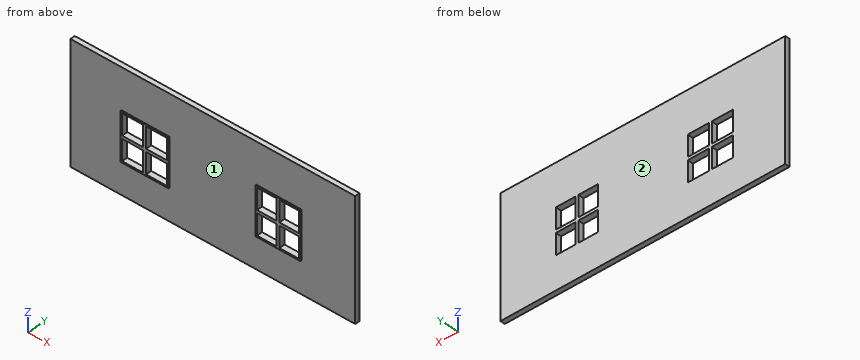
```python
from build123d import *

# Parameters (mm, degrees)
F0_W      = 95
F0_H      = 1.6
F1_DEPTH  = 40
F2_W      = 15
F2_H      = 15
F2_W_2    = 14
F3_DEPTH  = 25
F4_W      = 16
F4_H      = 16
F4_W_2    = 15
F4_H_2    = 15
F4_W_3    = 14
F5_DEPTH  = 0.3
F6_W      = 1
F6_H      = 1.9
F7_DEPTH  = 15
F11_DEPTH = 15
F10_W     = 1.9
F10_H     = 1
F12_DEPTH = 14


with BuildPart() as f1:
    # F0 (on Top) → F1 (new body)
    with BuildSketch(Plane.XY):
        Rectangle(F0_W, F0_H)
    extrude(amount=F1_DEPTH)

    # F2 (on face) → F3 (cut)
    with BuildSketch(Plane.XZ.offset(0.8)):
        with Locations((-22.5, 18.5)):
            Rectangle(F2_W, F2_H)
        with Locations((22, 18.5)):
            Rectangle(F2_W_2, F2_H)
    extrude(amount=-F3_DEPTH, mode=Mode.SUBTRACT)

    # F4 (on face) → F5 (join)
    with BuildSketch(Plane.XZ.offset(0.8)):
        with Locations((-22.5, 18.5)):
            Rectangle(F4_W, F4_H)
        with Locations((-22.5, 18.5)):
            Rectangle(F4_W_2, F4_H_2, mode=Mode.SUBTRACT)
        with Locations((22, 18.5)):
            Rectangle(F4_W_2, F4_H)
        with Locations((22, 18.5)):
            Rectangle(F4_W_3, F4_H_2, mode=Mode.SUBTRACT)
    extrude(amount=F5_DEPTH)

    # F6 (on face) → F7 (join, through all)
    with BuildSketch(Plane.XY.offset(11)):
        with Locations((22, -0.15)):
            Rectangle(F6_W, F6_H)
        with Locations((-22.5, -0.15)):
            Rectangle(F6_W, F6_H)
    extrude(amount=F7_DEPTH)

    # F9 (on face) → F11 (join, through all)
    with BuildSketch(Plane(origin=(-15, 0, 0), x_dir=(0, -1, 0), z_dir=(-1, 0, 0))):
        Polygon((-0.8, 18), (0.8, 18), (1.1, 18), (1.1, 19), (-0.8, 19), align=None)
    extrude(amount=F11_DEPTH)

    # F10 (on face) → F12 (join, through all)
    with BuildSketch(Plane(origin=(29, 0, 0), x_dir=(0, -1, 0), z_dir=(-1, 0, 0))):
        with Locations((0.15, 18.5)):
            Rectangle(F10_W, F10_H)
    extrude(amount=F12_DEPTH)


solid = f1.part
```
Read the model definition and answer for the solid it produces. Units are mm, in the model's axes. Face numbers are marked on the shaded views. Give positions to 0.01 mm unless a question says otherwise; leave off trailing zeros. Write each loop counter-clockwise with the first axis right and the second up, starting at its lowest first coordinate (ties: lowest second). Pieces come first, ordered by that corner, then holes. Notation, with made-up numbers: M 39,69 L 43,69 A22 ccw 43,93 Z; hole C -8.5,-6 d6. An arc over 180 degrees is marked long. Put each result on its own line as item: value. Start each with the question number.
1. The part is cut by section C-C, the plane y = 0.1. Give the number of separate pieces and of enclosed holes in the cut face, and give its area (3 significant figures).
2. Consider line 1 along Z through (x, y) = (19, 0.25); line 2 along X through (y, z) = (0.7, 22.5); line 3 along Y through (x, z) = (-41, 27). Determine where each line is inside the solid, lowest interval first.
3. For a pull along X with two mould halves and no side action, classify the marked faces 1 and 2 as released by +X, released by -X, zero draft, split by the parting line, or undercut.
4. The part is cut by section D-D, the plane x = 5.5. Give the vertices of the cut face in (y, z).
5. The part is cut by section B-B, the plane x = -18.5. Give the vertices of the cut face in (y, z), and give its area (3 significant figures).
6. The part is cut by section A-A, the plane z = 15.5. Give the vertices of the cut face in (x, y).
Final values:
1. separate pieces: 1
1. enclosed holes: 8
1. area: 3,420 mm²
2. line 1: z = 0 to 11, 18 to 19, 26 to 40
2. line 2: x = -47.5 to -30, -23 to -22, -15 to 15, 21.5 to 22.5, 29 to 47.5
2. line 3: y = -0.8 to 0.8
3. face 1: undercut
3. face 2: zero draft
4. outline: M -0.8,0 L 0.8,0 L 0.8,40 L -0.8,40 Z
5. outline: M -1.1,10.5 L -0.8,10.5 L -0.8,0 L 0.8,0 L 0.8,11 L -1.1,11 Z; M -1.1,18 L 0.8,18 L 0.8,19 L -1.1,19 Z; M -1.1,26 L 0.8,26 L 0.8,40 L -0.8,40 L -0.8,26.5 L -1.1,26.5 Z
5. area: 42.2 mm²
6. outline: M -47.5,-0.8 L -30.5,-0.8 L -30.5,-1.1 L -30,-1.1 L -30,0.8 L -47.5,0.8 Z; M -23,-1.1 L -22,-1.1 L -22,0.8 L -23,0.8 Z; M -15,-1.1 L -14.5,-1.1 L -14.5,-0.8 L 14.5,-0.8 L 14.5,-1.1 L 15,-1.1 L 15,0.8 L -15,0.8 Z; M 21.5,-1.1 L 22.5,-1.1 L 22.5,0.8 L 21.5,0.8 Z; M 29,-1.1 L 29.5,-1.1 L 29.5,-0.8 L 47.5,-0.8 L 47.5,0.8 L 29,0.8 Z
